Input: part model. Units: mm. Frame: model coordinates. Give positions to 0.01 mm unless a question says otherwise; leave off trailing zeros. Write each loop counter-clockwise with the first axis right and the second up, starting at its lowest first coordinate (ties: lowest second). Pieces come first, ordered by that corner, then holes. Notation, with made-up numbers: (53, 16) - (74, 16) arc R5 cw to (74, 22) - close; hole circle Ø11 at (70.25, -14). An arc over 180 degrees is marked (long way). Answer as CSV lines item,"result". Start each with the question number.
from build123d import *

# Parameters (mm, degrees)
F1_DEPTH = 2.54


with BuildPart() as f1:
    # F0 (on Front) → F1 (new body)
    with BuildSketch(Plane.XZ):
        with BuildLine():
            Line((-1.5875, 30.622215), (-3.036757, 25.213515))
            ThreePointArc((-3.036757, 25.213515), (-4.704564, 23.651443), (-6.843197, 24.456367))
            Line((-6.843197, 24.456367), (-10.251956, 28.898748))
            ThreePointArc((-10.251956, 28.898748), (-10.930814, 29.352346), (-11.745522, 29.298948))
            Line((-11.745522, 29.298948), (-12.078834, 29.160885))
            Line((-12.078834, 29.160885), (-12.412146, 29.022823))
            ThreePointArc((-12.412146, 29.022823), (-13.02599, 28.484496), (-13.185273, 27.683728))
            Line((-13.185273, 27.683728), (-12.454392, 22.132134))
            ThreePointArc((-12.454392, 22.132134), (-13.397466, 20.050725), (-15.681336, 19.975959))
            Line((-15.681336, 19.975959), (-20.530644, 22.775708))
            ThreePointArc((-20.530644, 22.775708), (-21.331412, 22.934991), (-22.06367, 22.573881))
            Line((-22.06367, 22.573881), (-22.318775, 22.318775))
            Line((-22.318775, 22.318775), (-22.573881, 22.06367))
            ThreePointArc((-22.573881, 22.06367), (-22.934991, 21.331412), (-22.775708, 20.530644))
            Line((-22.775708, 20.530644), (-19.975959, 15.681336))
            ThreePointArc((-19.975959, 15.681336), (-20.050725, 13.397466), (-22.132134, 12.454392))
            Line((-22.132134, 12.454392), (-27.683728, 13.185273))
            ThreePointArc((-27.683728, 13.185273), (-28.484496, 13.02599), (-29.022823, 12.412146))
            Line((-29.022823, 12.412146), (-29.160885, 12.078834))
            Line((-29.160885, 12.078834), (-29.298948, 11.745522))
            ThreePointArc((-29.298948, 11.745522), (-29.352346, 10.930814), (-28.898748, 10.251956))
            Line((-28.898748, 10.251956), (-24.456367, 6.843197))
            ThreePointArc((-24.456367, 6.843197), (-23.651443, 4.704564), (-25.213515, 3.036757))
            Line((-25.213515, 3.036757), (-30.622215, 1.5875))
            ThreePointArc((-30.622215, 1.5875), (-31.301074, 1.133901), (-31.563515, 0.360774))
            Line((-31.563515, 0.360774), (-31.563515, 0))
            Line((-31.563515, 0), (-31.563515, -0.360774))
            ThreePointArc((-31.563515, -0.360774), (-31.301074, -1.133901), (-30.622215, -1.5875))
            Line((-30.622215, -1.5875), (-25.213515, -3.036757))
            ThreePointArc((-25.213515, -3.036757), (-23.651443, -4.704564), (-24.456367, -6.843197))
            Line((-24.456367, -6.843197), (-28.898748, -10.251956))
            ThreePointArc((-28.898748, -10.251956), (-29.352346, -10.930814), (-29.298948, -11.745522))
            Line((-29.298948, -11.745522), (-29.160885, -12.078834))
            Line((-29.160885, -12.078834), (-29.022823, -12.412146))
            ThreePointArc((-29.022823, -12.412146), (-28.484496, -13.02599), (-27.683728, -13.185273))
            Line((-27.683728, -13.185273), (-22.132134, -12.454392))
            ThreePointArc((-22.132134, -12.454392), (-20.050725, -13.397466), (-19.975959, -15.681336))
            Line((-19.975959, -15.681336), (-22.775708, -20.530644))
            ThreePointArc((-22.775708, -20.530644), (-22.934991, -21.331412), (-22.573881, -22.06367))
            Line((-22.573881, -22.06367), (-22.318775, -22.318775))
            Line((-22.318775, -22.318775), (-22.06367, -22.573881))
            ThreePointArc((-22.06367, -22.573881), (-21.331412, -22.934991), (-20.530644, -22.775708))
            Line((-20.530644, -22.775708), (-15.681336, -19.975959))
            ThreePointArc((-15.681336, -19.975959), (-13.397466, -20.050725), (-12.454392, -22.132134))
            Line((-12.454392, -22.132134), (-13.185273, -27.683728))
            ThreePointArc((-13.185273, -27.683728), (-13.02599, -28.484496), (-12.412146, -29.022823))
            Line((-12.412146, -29.022823), (-12.078834, -29.160885))
            Line((-12.078834, -29.160885), (-11.745522, -29.298948))
            ThreePointArc((-11.745522, -29.298948), (-10.930814, -29.352346), (-10.251956, -28.898748))
            Line((-10.251956, -28.898748), (-6.843197, -24.456367))
            ThreePointArc((-6.843197, -24.456367), (-4.704564, -23.651443), (-3.036757, -25.213515))
            Line((-3.036757, -25.213515), (-1.5875, -30.622215))
            ThreePointArc((-1.5875, -30.622215), (-1.133901, -31.301074), (-0.360774, -31.563515))
            Line((-0.360774, -31.563515), (0, -31.563515))
            Line((0, -31.563515), (0.360774, -31.563515))
            ThreePointArc((0.360774, -31.563515), (1.133901, -31.301074), (1.5875, -30.622215))
            Line((1.5875, -30.622215), (3.036757, -25.213515))
            ThreePointArc((3.036757, -25.213515), (4.704564, -23.651443), (6.843197, -24.456367))
            Line((6.843197, -24.456367), (10.251956, -28.898748))
            ThreePointArc((10.251956, -28.898748), (10.930814, -29.352346), (11.745522, -29.298948))
            Line((11.745522, -29.298948), (12.078834, -29.160885))
            Line((12.078834, -29.160885), (12.412146, -29.022823))
            ThreePointArc((12.412146, -29.022823), (13.02599, -28.484496), (13.185273, -27.683728))
            Line((13.185273, -27.683728), (12.454392, -22.132134))
            ThreePointArc((12.454392, -22.132134), (13.397466, -20.050725), (15.681336, -19.975959))
            Line((15.681336, -19.975959), (20.530644, -22.775708))
            ThreePointArc((20.530644, -22.775708), (21.331412, -22.934991), (22.06367, -22.573881))
            Line((22.06367, -22.573881), (22.318775, -22.318775))
            Line((22.318775, -22.318775), (22.573881, -22.06367))
            ThreePointArc((22.573881, -22.06367), (22.934991, -21.331412), (22.775708, -20.530644))
            Line((22.775708, -20.530644), (19.975959, -15.681336))
            ThreePointArc((19.975959, -15.681336), (20.050725, -13.397466), (22.132134, -12.454392))
            Line((22.132134, -12.454392), (27.683728, -13.185273))
            ThreePointArc((27.683728, -13.185273), (28.484496, -13.02599), (29.022823, -12.412146))
            Line((29.022823, -12.412146), (29.160885, -12.078834))
            Line((29.160885, -12.078834), (29.298948, -11.745522))
            ThreePointArc((29.298948, -11.745522), (29.352346, -10.930814), (28.898748, -10.251956))
            Line((28.898748, -10.251956), (24.456367, -6.843197))
            ThreePointArc((24.456367, -6.843197), (23.651443, -4.704564), (25.213515, -3.036757))
            Line((25.213515, -3.036757), (30.622215, -1.5875))
            ThreePointArc((30.622215, -1.5875), (31.301074, -1.133901), (31.563515, -0.360774))
            Line((31.563515, -0.360774), (31.563515, 0))
            Line((31.563515, 0), (31.563515, 0.360774))
            ThreePointArc((31.563515, 0.360774), (31.301074, 1.133901), (30.622215, 1.5875))
            Line((30.622215, 1.5875), (25.213515, 3.036757))
            ThreePointArc((25.213515, 3.036757), (23.651443, 4.704564), (24.456367, 6.843197))
            Line((24.456367, 6.843197), (28.898748, 10.251956))
            ThreePointArc((28.898748, 10.251956), (29.352346, 10.930814), (29.298948, 11.745522))
            Line((29.298948, 11.745522), (29.160885, 12.078834))
            Line((29.160885, 12.078834), (29.022823, 12.412146))
            ThreePointArc((29.022823, 12.412146), (28.484496, 13.02599), (27.683728, 13.185273))
            Line((27.683728, 13.185273), (22.132134, 12.454392))
            ThreePointArc((22.132134, 12.454392), (20.050725, 13.397466), (19.975959, 15.681336))
            Line((19.975959, 15.681336), (22.775708, 20.530644))
            ThreePointArc((22.775708, 20.530644), (22.934991, 21.331412), (22.573881, 22.06367))
            Line((22.573881, 22.06367), (22.318775, 22.318775))
            Line((22.318775, 22.318775), (22.06367, 22.573881))
            ThreePointArc((22.06367, 22.573881), (21.331412, 22.934991), (20.530644, 22.775708))
            Line((20.530644, 22.775708), (15.681336, 19.975959))
            ThreePointArc((15.681336, 19.975959), (13.397466, 20.050725), (12.454392, 22.132134))
            Line((12.454392, 22.132134), (13.185273, 27.683728))
            ThreePointArc((13.185273, 27.683728), (13.02599, 28.484496), (12.412146, 29.022823))
            Line((12.412146, 29.022823), (12.078834, 29.160885))
            Line((12.078834, 29.160885), (11.745522, 29.298948))
            ThreePointArc((11.745522, 29.298948), (10.930814, 29.352346), (10.251956, 28.898748))
            Line((10.251956, 28.898748), (6.843197, 24.456367))
            ThreePointArc((6.843197, 24.456367), (4.704564, 23.651443), (3.036757, 25.213515))
            Line((3.036757, 25.213515), (1.5875, 30.622215))
            ThreePointArc((1.5875, 30.622215), (1.133901, 31.301074), (0.360774, 31.563515))
            Line((0.360774, 31.563515), (0, 31.563515))
            Line((0, 31.563515), (-0.360774, 31.563515))
            ThreePointArc((-0.360774, 31.563515), (-1.133901, 31.301074), (-1.5875, 30.622215))
        make_face()
    extrude(amount=F1_DEPTH)


solid = f1.part
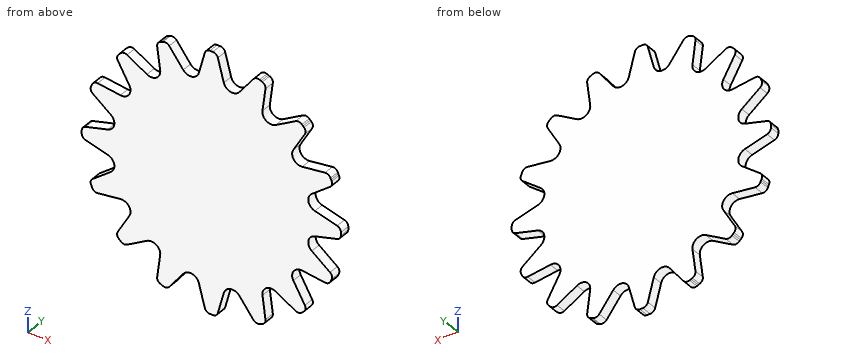
1) Contact query for flat-ended pins moving along their axis: P1, Ø1.5, axis at x = 17, y = -1.5, coming from the -Z side; P2, Ø1, axis at x = 12, y = -1, coming from the -Z side. Output: stop coordinate, or through.
2) Cut plane A-A on z = -26. Output: boundary loops of the cut face in (x, y), and give its area (3 significant figures).
3) Material intervals for line 1 (X direction, y = -0.45, z = -24); line 2 (Z direction, x = -13.5, y = -1.4); line 3 (X direction, y = -0.4, z = -27) (3 decimals), sorted ascending. Write a range as from..to.
4) Cut plane C-C on z = 6. Output: boundary loops of the cut face in (x, y), and give its area (3 significant figures).
5) Cut plane B-B on x = -14. Output: boundary loops of the cut face in (y, z), and give its area (3 significant figures).
Numbers:
1,P1,"stops at z = -21.17"
1,P2,"stops at z = -29.37"
2,outline,"(-12.96, -2.54) - (-8.03, -2.54) - (-8.03, 0) - (-12.96, 0) - close; (-2.83, -2.54) - (2.83, -2.54) - (2.83, 0) - (-2.83, 0) - close; (8.03, -2.54) - (12.96, -2.54) - (12.96, 0) - (8.03, 0) - close"
2,area,"39.4 mm²"
3,line 1,"x = -12.7..-6.37, -3.89..3.89, 6.37..12.7"
3,line 2,"z = -19.99..19.99"
3,line 3,"x = -13.095..-8.795, -2.558..2.558, 8.795..13.095"
4,outline,"(-23.79, -2.54) - (23.79, -2.54) - (23.79, 0) - (-23.79, 0) - close"
4,area,"121 mm²"
5,outline,"(-2.54, -19.77) - (0, -19.77) - (0, 19.77) - (-2.54, 19.77) - close"
5,area,"100 mm²"
